Work out the finished part from the listing and answer in its coordinate system (mm). Face numbers are marked on the shaded views. A direction names the side the tool comes from. Coordinates: 2 decimals unless noted, no trailing zeros. Loops run counter-clockwise (first coordinate to the right, second up) from the corner with the lowest first, then second, coordinate; pieces in that order, holes last. Notation, with made-up numbers: M 23.25,45.5 L 27.25,45.5 A22 cw 27.25,65.5 Z; hole C 82.25,10 d6. An arc over 180 degrees is marked long. Write each question's results on one line, items separated by ' | '.
```python
from build123d import *

# Parameters (mm, degrees)
CROQUIS1_R                 = 9.5
SALIENTE_EXTRUIR1_DEPTH    = 25
SALIENTE_EXTRUIR2_DEPTH    = 3
CORTAR_EXTRUIR1_DEPTH      = 42.880783183
CORTAR_EXTRUIR1_DEPTH_BACK = 200
CROQUIS3_R                 = 2.6
CROQUIS4_R                 = 4.5
CORTAR_EXTRUIR2_DEPTH      = 10
CORTAR_EXTRUIR3_DEPTH      = 10
CORTAR_EXTRUIR3_DEPTH_BACK = 10
CROQUIS5_R                 = 2
CORTAR_EXTRUIR4_DEPTH      = 0.5
CORTAR_EXTRUIR4_DEPTH_BACK = 10.5
CROQUIS6_R                 = 4.5


with BuildPart() as part:
    # Croquis1 → Saliente-Extruir1 (new body)
    with BuildSketch(Plane.XY):
        with BuildLine():
            Line((0, 13.5), (-20, 13.5))
            Line((-20, 13.5), (-20, 3.5))
            ThreePointArc((-20, 3.5), (-13.124404748, -8.675770292), (0, -13.5))
            ThreePointArc((0, -13.5), (13.124404748, -8.675770292), (20, 3.5))
            Line((20, 3.5), (20, 13.5))
            Line((20, 13.5), (0, 13.5))
        make_face()
        Circle(CROQUIS1_R, mode=Mode.SUBTRACT)
    extrude(amount=SALIENTE_EXTRUIR1_DEPTH)

    # Croquis2 → Saliente-Extruir2 (add)
    with BuildSketch(Plane(origin=(0, 0, 0), x_dir=(-1, 0, 0), z_dir=(0, 0, -1))):
        with BuildLine():
            Line((20, 13.5), (-20, 13.5))
            Line((-20, 13.5), (-20, 3.5))
            ThreePointArc((-20, 3.5), (0, -13.5), (20, 3.5))
            Line((20, 3.5), (20, 13.5))
        make_face()
    extrude(amount=-SALIENTE_EXTRUIR2_DEPTH)

    # Croquis3 → Cortar-Extruir1 (cut, two sides: drawn at the far end of the back side and taken through both)
    with BuildSketch(Plane(origin=(0, 13.5, 0), x_dir=(1, 0, 0), z_dir=(0, 1, 0)).offset(-CORTAR_EXTRUIR1_DEPTH_BACK)):
        with Locations((14.75, -12.5)):
            Circle(CROQUIS3_R)
        with Locations((-14.75, -12.5)):
            Circle(CROQUIS3_R)
    extrude(amount=CORTAR_EXTRUIR1_DEPTH + CORTAR_EXTRUIR1_DEPTH_BACK, mode=Mode.SUBTRACT)

    # Croquis4 → Cortar-Extruir2 (cut)
    with BuildSketch(Plane(origin=(0, -11.5, 0), x_dir=(1, 0, 0), z_dir=(0, 1, 0))):
        with Locations((-14.75, -12.5)):
            Circle(CROQUIS4_R)
        with Locations((14.75, -12.5)):
            Circle(CROQUIS4_R)
    extrude(amount=CORTAR_EXTRUIR2_DEPTH, mode=Mode.SUBTRACT)

    # Croquis5 → Cortar-Extruir3 (cut, two sides: drawn at the far end of the back side and taken through both)
    with BuildSketch(Plane(origin=(0, -11.5, 0), x_dir=(1, 0, 0), z_dir=(0, 1, 0)).offset(-CORTAR_EXTRUIR3_DEPTH_BACK)):
        with Locations(Location((0, -12.5, 0), (0, 0, 180))):
            Circle(CROQUIS5_R)
    extrude(amount=CORTAR_EXTRUIR3_DEPTH + CORTAR_EXTRUIR3_DEPTH_BACK, mode=Mode.SUBTRACT)

    # Croquis6 → Cortar-Extruir4 (cut, two sides: drawn at the far end of the back side and taken through both)
    with BuildSketch(Plane(origin=(0, -11.5, 0), x_dir=(1, 0, 0), z_dir=(0, 1, 0)).offset(-CORTAR_EXTRUIR4_DEPTH_BACK)):
        with Locations((0, -12.5)):
            Circle(CROQUIS6_R)
    extrude(amount=CORTAR_EXTRUIR4_DEPTH + CORTAR_EXTRUIR4_DEPTH_BACK, mode=Mode.SUBTRACT)


solid = part.part
```
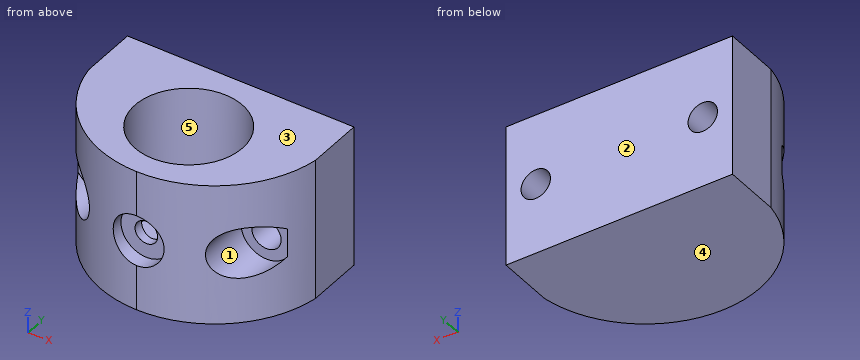
1) Given pin 1 Ø8 at (x, z) = (0, 12.5) entering from -Y; pin 2 Ø8 at (y, z) = (-1, 9.5) entering from +X; pin 3 Ø11.5 at (x, y) = (0, 0) entering from +Z, each flat-ended and moving along its own axis, determine where each tip first touches the part or whether it passes through.
Check result:
pin 1: y = -11 | pin 2: x = 19.91 | pin 3: z = 3
2) Straight lines are drawn through the part: probe 1 along X at (y, z) = (1, 12.75); probe 2 along Z at (x, y) = (14.75, -6.25); probe 3 along Y at (x, z) = (-11, 17.25). For each, find the intervals that lie inside material, in ascending order. Write a range as [from, to].
Check result:
probe 1: [-19.43, -17.34], [-12.16, -9.45], [9.45, 12.16], [17.34, 19.43] | probe 2: [0, 8], [17, 25] | probe 3: [-10.25, 13.5]
3) Find section C-C, the plane z = 15.75. Give the vertices of the cut face in (x, y), and give its area (3 significant figures).
Check result:
outline: M -20,3.5 A20.26 ccw -17.86,-2.81 L -17.86,-1.5 L -11.64,-1.5 L -11.64,-9.83 A20.26 ccw -3.11,-13.26 L -3.11,-11 L 3.11,-11 L 3.11,-13.26 A20.26 ccw 11.64,-9.83 L 11.64,-1.5 L 17.86,-1.5 L 17.86,-2.81 A20.26 ccw 20,3.5 L 20,13.5 L -20,13.5 Z; hole C 0,0 d19 | area: 548 mm^2
4) For a pull along Z with two mould halves and no side action, classify the marked faces 1, 2 and 3 as released by +Z, released by -Z, zero draft, split by the parting line, or undercut.
Check result:
face 1: undercut | face 2: zero draft | face 3: released by +Z
5) Find section A-A, the plane x = 14.75. Give the vertices of the cut face in (y, z), and give its area (3 significant figures).
Check result:
outline: M -7.13,0 L 13.5,0 L 13.5,9.9 L -1.5,9.9 L -1.5,8 L -7.13,8 Z; M -7.13,17 L -1.5,17 L -1.5,15.1 L 13.5,15.1 L 13.5,25 L -7.13,25 Z | area: 387 mm^2
6) Find section B-B, the plane y = 7.75. Give the vertices of the cut face in (x, z).
Check result:
outline: M -20,0 L 20,0 L 20,25 L 5.49,25 L 5.49,3 L -5.49,3 L -5.49,25 L -20,25 Z; hole C -14.75,12.5 d5.2; hole C 14.75,12.5 d5.2
7) Find section D-D, the plane z = 12.5. Give the vertices of the cut face in (x, y), and give its area (3 significant figures).
Check result:
outline: M -20,3.5 A20.26 ccw -18.5,-1.5 L -17.35,-1.5 L -17.35,13.5 L -20,13.5 Z; M -12.15,-1.5 L -10.25,-1.5 L -10.25,-10.72 A20.26 ccw -4.5,-12.99 L -4.5,-11 L -2,-11 L -2,-9.29 A9.5 cw long 2,-9.29 L 2,-11 L 4.5,-11 L 4.5,-12.99 A20.26 ccw 10.25,-10.72 L 10.25,-1.5 L 12.15,-1.5 L 12.15,13.5 L -12.15,13.5 Z; M 17.35,-1.5 L 18.5,-1.5 A20.26 ccw 20,3.5 L 20,13.5 L 17.35,13.5 Z | area: 354 mm^2
8) Which of the six approach directions +Z, -Z, +X, -X, +Y, -Y give full straight-line access (tool end or side, diameter ignored) to the marked faces 4 and 5?
Check result:
face 4: -Z, +X, -X, +Y, -Y | face 5: +Z
